Read the model definition and answer for the solid it produces. Units are mm, in the model's axes. A direction names the side the tool comes from. Coordinates: 2 decimals unless noted, no trailing zeros. Order: outer loops, then holes, each group sorted by start corner. A loop starts at its lowest first (then second) coordinate and runs counter-clockwise, first axis right, second up. Notation, with made-up numbers: M 2,-13.75 L 47,-13.75 A34 ccw 47,19.25 Z; hole C -33,19 d5. An arc over 180 degrees is marked long. Write each question's results on one line, items separated by ' | '.
```python
from build123d import *

# Parameters (mm, degrees)
F0_W     = 10.25
F0_H     = 10.25
F0_W_2   = 6.25
F0_H_2   = 6.25
F1_DEPTH = 4.5
F2_R     = 1
F3_R     = 0.5


with BuildPart() as f1:
    # F0 (on Top) → F1 (new body)
    with BuildSketch(Plane.XY):
        with Locations((3.125, 3.125)):
            Rectangle(F0_W, F0_H)
        with Locations((3.125, 3.125)):
            Rectangle(F0_W_2, F0_H_2, mode=Mode.SUBTRACT)
    extrude(amount=F1_DEPTH)

    # F2
    f2_edges = [f1.edges().sort_by_distance(p)[0] for p in [
        (-2, -2, 2.25),
        (8.25, -2, 2.25),
        (8.25, 8.25, 2.25),
        (-2, 8.25, 2.25),
    ]]
    fillet(f2_edges, radius=F2_R)

    # F3
    f3_edges = [f1.edges().sort_by_distance(p)[0] for p in [
        (0, 6.25, 2.25),
        (6.25, 6.25, 2.25),
        (0, 0, 2.25),
        (6.25, 0, 2.25),
    ]]
    fillet(f3_edges, radius=F3_R)


solid = f1.part
```
(1) The part is cut by section D-D, the plane y = 7.75. Write down the section's boundary in (x, z), then the cut area to 3 significant figures.
Conclusion:
outline: M -1.87,0 L 8.12,0 L 8.12,4.5 L -1.87,4.5 Z | area: 44.9 mm²
(2) The part is cut by section A-A, the plane x = 5.5. Write down the section's boundary in (y, z), then the cut area to 3 significant figures.
Conclusion:
outline: M -2,0 L 0,0 L 0,4.5 L -2,4.5 Z; M 6.25,0 L 8.25,0 L 8.25,4.5 L 6.25,4.5 Z | area: 18.0 mm²
(3) The part is cut by section B-B, the plane z = 2.95. Write down the section's boundary in (x, y), then the cut area to 3 significant figures.
Conclusion:
outline: M -2,-1 A1 ccw -1,-2 L 7.25,-2 A1 ccw 8.25,-1 L 8.25,7.25 A1 ccw 7.25,8.25 L -1,8.25 A1 ccw -2,7.25 Z; hole M 0,0.5 A0.5 ccw 0.5,0 L 5.75,0 A0.5 ccw 6.25,0.5 L 6.25,5.75 A0.5 ccw 5.75,6.25 L 0.5,6.25 A0.5 ccw 0,5.75 Z | area: 65.4 mm²
(4) Straight lines are drawn through the part: line 1 (Y direction, x = 5.5, z = 2.3); line 2 (X direction, y = 6, z = 1.95). For each, find the intervals that lie inside material, in ascending order.
Conclusion:
line 1: -2 to 0, 6.25 to 8.25 | line 2: -2 to 0.07, 6.18 to 8.25
(5) For faces 5 (the flat face through (6.25, 3, 2)), 6 (the flat face through (3, -2, 2)), determine the directions among +Z, -Z, +X, -X, +Y, -Y from which every point of the face is accessible in a straight line to the end or side of a thin tool.
Conclusion:
face 5: +Z, -Z | face 6: +Z, -Z, +X, -X, -Y
(6) The mould has two halves that part along X. Classify faces 1 (the flat face through (3, 6.25, 2)), 2 (the flat face through (3, 7, 0)), 3 (the cylindrical face through (-1.715, -1.699, 2.282)), 4 (the flat face through (3, 0, 2)): pulls with the +X half, pulls with the -X half, needs draft (parallel to the pull), parting line crosses it, or undercut.
Conclusion:
face 1: undercut | face 2: needs draft | face 3: pulls with the -X half | face 4: undercut
